Can you work these out from the model? Positions are in its coordinate system, mm. Face numbers are marked on the shaded views. Round coordinates to 2 decimals unless told otherwise and drop trailing zeros. Loops run counter-clockwise (first coordinate to the right, second up) from the corner with the lowest first, then second, coordinate; pieces in that order, holes last. Notation, with made-up numbers: M 27.25,30.5 L 71.25,30.5 A30 cw 71.25,57.5 Z; hole C 11,33 d5. An arc over 180 degrees is marked long. Answer as CSV lines item,"result".
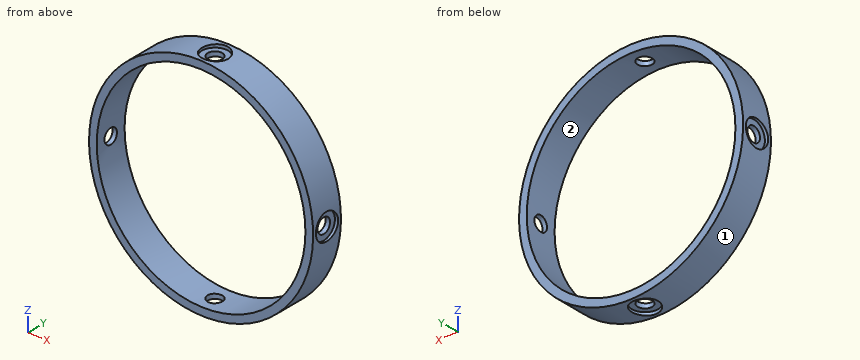
from build123d import *

# Parameters (mm, degrees)
SKETCH1_R               = 34.1
SKETCH1_R_2             = 31.75
BOSS_EXTRUDE1_DEPTH     = 5
SKETCH2_R               = 4
CUT_EXTRUDE1_DEPTH      = 1
CUT_EXTRUDE2_REACH      = 77.523
CUT_EXTRUDE2_END_RADIUS = 31.75
SKETCH3_R               = 2.25
CIRPATTERN1_COUNT       = 4


with BuildPart() as part:
    # Sketch1 → Boss-Extrude1 (new, symmetric)
    with BuildSketch(Plane(origin=(0, 0, 0), x_dir=(1, 0, 0), z_dir=(0, 1, 0))):
        with Locations(Location((0, 0, 0), (0, 0, 270))):
            Circle(SKETCH1_R)
        with Locations(Location((0, 0, 0), (0, 0, 270))):
            Circle(SKETCH1_R_2, mode=Mode.SUBTRACT)
    extrude(amount=BOSS_EXTRUDE1_DEPTH, both=True)

    # Sketch2 → Cut-Extrude1 (cut)
    with BuildSketch(Plane(origin=(0, 0, -34.1), x_dir=(-1, 0, 0), z_dir=(0, 0, -1))):
        Circle(SKETCH2_R)
    cut_extrude1 = extrude(amount=-CUT_EXTRUDE1_DEPTH, mode=Mode.SUBTRACT)

    # Cut-Extrude2: up to this cylinder (the profile starts outside it)
    cut_extrude2_end = Plane(origin=(0, 0, 0), z_dir=(0, -1, 0)) * Cylinder(CUT_EXTRUDE2_END_RADIUS, 219.546, mode=Mode.PRIVATE)
    # Sketch3 → Cut-Extrude2 (cut, up to the surface)
    with BuildSketch(Plane(origin=(0, 0, -33.1), x_dir=(-1, 0, 0), z_dir=(0, 0, -1)), mode=Mode.PRIVATE) as cut_extrude2_sk1:
        Circle(SKETCH3_R)
    cut_extrude2_tool1 = extrude(cut_extrude2_sk1.sketch, amount=-CUT_EXTRUDE2_REACH, mode=Mode.PRIVATE) - cut_extrude2_end
    cut_extrude2 = cut_extrude2_tool1.solids().sort_by_distance((0, 0, -33.1))[0]
    add(cut_extrude2, mode=Mode.SUBTRACT)

    # CirPattern1: Cut-Extrude1, Cut-Extrude2 ×4 about axis
    cirpattern1_axis = Axis((0, 0, 0), (0, 1, 0))
    add([cut_extrude1.rotate(cirpattern1_axis, i * 360 / CIRPATTERN1_COUNT) for i in range(1, CIRPATTERN1_COUNT)], mode=Mode.SUBTRACT)
    add([cut_extrude2.rotate(cirpattern1_axis, i * 360 / CIRPATTERN1_COUNT) for i in range(1, CIRPATTERN1_COUNT)], mode=Mode.SUBTRACT)


solid = part.part
Item 1: Will these pins go through, and if not, where does the flat tip stop? pin 1 (5 mm diameter, centred on x = 0, y = 0, fed in from -Z); pin 2 (1 mm diameter, centred on y = 1.5, z = 20, fed in from +X); pin 3 (2 mm diameter, centred on y = 3.5, z = -25.5, fed in from -X).
Output:
pin 1,"stops at z = -33.1"
pin 2,"stops at x = 27.97"
pin 3,"stops at x = -23.72"
Item 2: If we section it at B-B on z = -12: Write out the boundary of the cut face in (x, y), then the cut area to 3 significant figures.
Output:
outline,"M -31.92,-5 L -29.39,-5 L -29.39,5 L -31.92,5 Z; M 29.39,-5 L 31.92,-5 L 31.92,5 L 29.39,5 Z"
area,"50.5 mm2"
Item 3: We'd pull the mould along Z, two halves only. Please class the marked faces 1 and 2: released by +Z, released by -Z, zero draft, split by the parting line, or undercut.
Output:
face 1,"split by the parting line"
face 2,"undercut"
Item 4: If we section it at C-C on y = 0: State how many separate pieces and enclosed holes the cut face has, then the cut area to 3 significant figures.
Output:
separate pieces,"4"
enclosed holes,"0"
area,"432 mm2"
Item 5: If I drill on line 1 along X through (y, z) = (2.75, 0); line 2 along X through (y, z) = (4, 12.5); line 3 along Y through (x, z) = (0, 32.65), over which ranges is the centre line in solid material (lowest first)? Write a range as from..to.
Output:
line 1,"x = -33.1..-31.75, 31.75..33.1"
line 2,"x = -31.73..-29.19, 29.19..31.73"
line 3,"y = -5..-2.25, 2.25..5"
Item 6: If we section it at D-D on z = 0: Write out the boundary of the cut face in (x, y), then the cut area to 4 significant figures.
Output:
outline,"M -34.1,-5 L -31.75,-5 L -31.75,-2.25 L -33.1,-2.25 L -33.1,-4 L -34.1,-4 Z; M -34.1,4 L -33.1,4 L -33.1,2.25 L -31.75,2.25 L -31.75,5 L -34.1,5 Z; M 31.75,-5 L 34.1,-5 L 34.1,-4 L 33.1,-4 L 33.1,-2.25 L 31.75,-2.25 Z; M 31.75,2.25 L 33.1,2.25 L 33.1,4 L 34.1,4 L 34.1,5 L 31.75,5 Z"
area,"18.85 mm2"
Item 7: If we section it at A-A on x = 0: Write out the boundary of the cut face in (y, z).
Output:
outline,"M -5,-34.1 L -4,-34.1 L -4,-33.1 L -2.25,-33.1 L -2.25,-31.75 L -5,-31.75 Z; M -5,31.75 L -2.25,31.75 L -2.25,33.1 L -4,33.1 L -4,34.1 L -5,34.1 Z; M 2.25,-33.1 L 4,-33.1 L 4,-34.1 L 5,-34.1 L 5,-31.75 L 2.25,-31.75 Z; M 2.25,31.75 L 5,31.75 L 5,34.1 L 4,34.1 L 4,33.1 L 2.25,33.1 Z"
